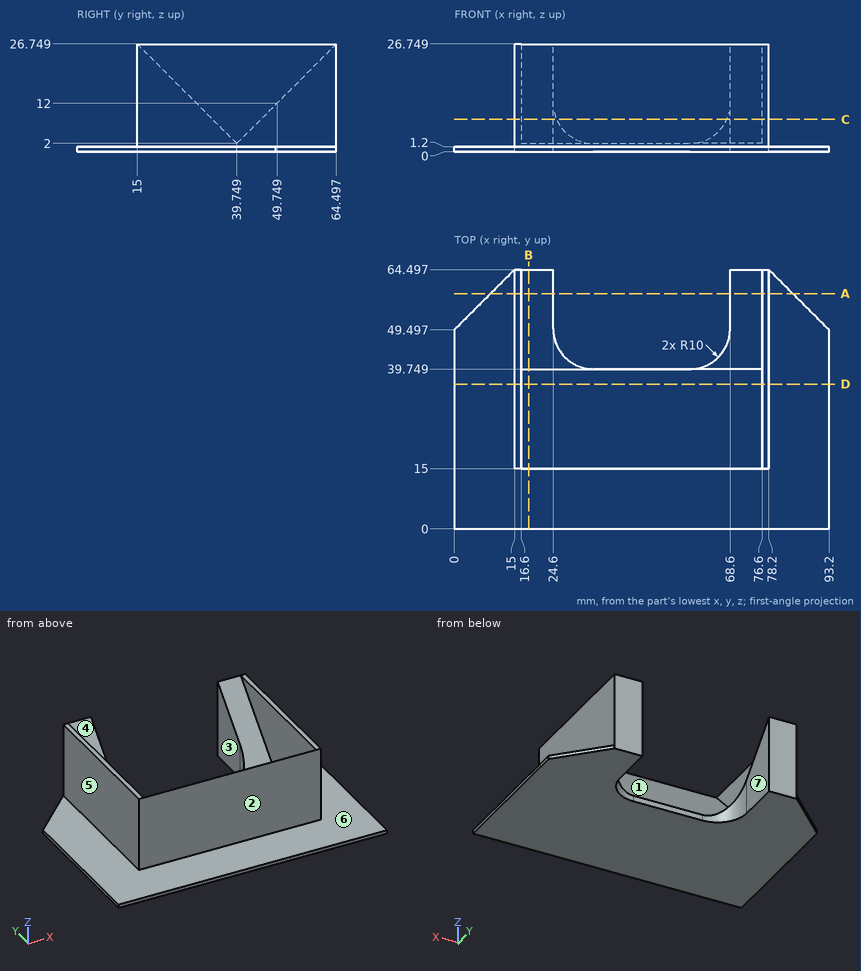
Input: dimensioned drawing with shaded views. Units: mm. Origin: part minimum x, y, z. A direction names the side the tool comes from. Coordinates: 2 decimals unless noted, no trailing zeros. Loops run counter-clockwise (first coordinate to the right, second up) from the corner with the lowest first, then second, coordinate; pieces in that order, holes last. Notation, with made-up numbers: M 81,2.25 L 140,2.25 A34 ccw 140,39.25 Z; hole C -20,-1.75 d1. An arc over 180 degrees is marked long. One line per item, written item: value. Start each with the question number.
1) Cut plane C-C (z = 8). Return loops of the section in (x, y) (1 decimal).
2) Cut plane A-A (y = 58.5). Return loops of the section in (x, z).
3) Pin query (flat end, axial travel): P1, Ø10, axis at y = 44.5, z = 16, coming from the +X side; P2, Ø6, axis at x = 66, z = 19.5, coming from the -Y side; P3, Ø0.6, axis at x = 51.5, z = 0.5, coming from the +Y side. Return the tip coordinate at first contact, or that it passes through.
4) Reachability of the marked faces 1, 2 and 3 from +Z, -Z, +X, -X, +Y, -Y: full face, straight path, thin tool, end or side. Return the list, or none.
5) Cut plane B-B (x = 18.5). Return loops of the section in (y, z).
6) Cut plane D-D (y = 36). Return loops of the section in (x, z).
7) Material intervals for L1, parallel to X at y = 43, z = 15; L2, parallel to Z at x = 63.5, y = 4.5; L3, parallel to X at y = 23, z = 2.5, sorted ascending. Write a range as from..to.
8) Draft query along X for the marked faces 4, 5, 6 and 7. Return one class per face: released by +X, released by -X, zero draft, split by the parting line, or undercut.
Evaluation:
1. outline: M 15,15 L 78.2,15 L 78.2,64.5 L 68.6,64.5 L 68.6,49.7 A10 cw 67.8,45.7 L 76.6,45.7 L 76.6,33.7 L 16.6,33.7 L 16.6,45.7 L 25.4,45.7 A10 cw 24.6,49.7 L 24.6,64.5 L 15,64.5 Z
2. outline: M 9,0 L 24.6,0 L 24.6,20.75 L 16.6,20.75 L 16.6,26.75 L 15,26.75 L 15,1.2 L 9,1.2 Z; M 68.6,0 L 84.2,0 L 84.2,1.2 L 78.2,1.2 L 78.2,26.75 L 76.6,26.75 L 76.6,20.75 L 68.6,20.75 Z
3. P1: x = 78.2
3. P2: y = 15
3. P3: y = 39.75
4. face 1: +Z
4. face 2: +Z, +X, -X, -Y
4. face 3: +Z, -Z, +Y
5. outline: M 0,0 L 64.5,0 L 64.5,26.75 L 39.75,2 L 15,26.75 L 15,1.2 L 0,1.2 Z
6. outline: M 0,0 L 93.2,0 L 93.2,1.2 L 78.2,1.2 L 78.2,26.75 L 76.6,26.75 L 76.6,5.75 L 16.6,5.75 L 16.6,26.75 L 15,26.75 L 15,1.2 L 0,1.2 Z
7. L1: 15..16.6, 76.6..78.2
7. L2: 0..1.2
7. L3: 15..78.2
8. face 4: undercut
8. face 5: released by -X
8. face 6: zero draft
8. face 7: undercut
